Can you work these out from the drawing? Everything is in mm from the part's minimum corner. Round coordinates to 2 decimals unless told otherwise and drop trailing zeros. Loops run counter-clockwise (first coordinate to the right, second up) from the corner with the lowest first, then second, coordinate; pieces in that order, holes last. Notation, with made-up numbers: (24, 80.5) - (69, 80.5) arc R21 ccw to (69, 98.5) - close; hole circle Ø10 at (-27, 45.5). An arc over 180 degrees is marked (long way). Answer as a JSON object with one key per item and string values. Group by question number.
1) I want a section at C-C, the plane y = 28. Please give me the cut outline in (x, z).
2) I want a section at B-B, the plane x = 1.1. Please give me the cut outline in (y, z).
3) I want a section at A-A, the plane z = 27. Please give me the cut outline in (x, y).
4) If I drill on line 1 along Y through (x, z) = (0.5, 3); line 2 along Z through (x, y) = (0.3, 3.5); line 3 along Y through (x, z) = (0.15, 28.5), over which ranges is the centre line in solid material (lowest first)? Write a range as [from, to].
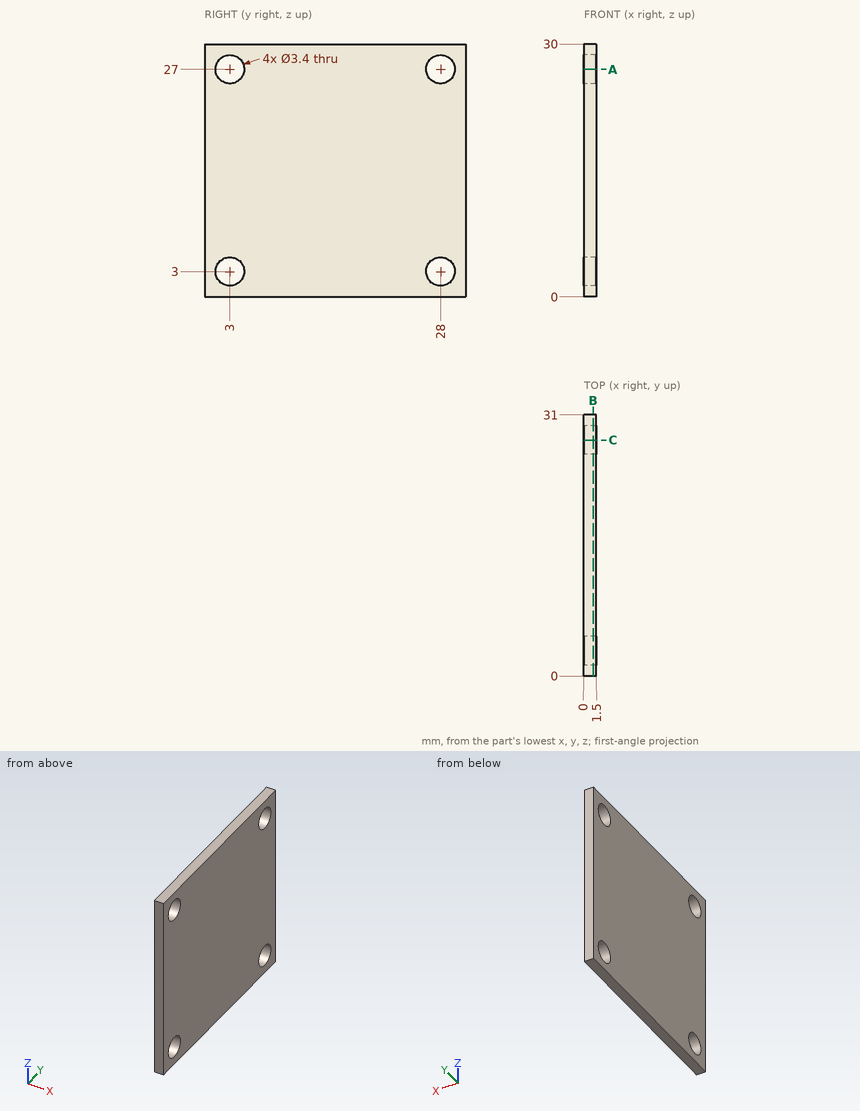
Outcome:
{
 "1": {"outline": "(0, 0) - (1.5, 0) - (1.5, 1.3) - (0, 1.3) - close; (0, 4.7) - (1.5, 4.7) - (1.5, 25.3) - (0, 25.3) - close; (0, 28.7) - (1.5, 28.7) - (1.5, 30) - (0, 30) - close"},
 "2": {"outline": "(0, 0) - (31, 0) - (31, 30) - (0, 30) - close; hole circle Ø3.4 at (3, 3); hole circle Ø3.4 at (3, 27); hole circle Ø3.4 at (28, 3); hole circle Ø3.4 at (28, 27)"},
 "3": {"outline": "(0, 0) - (1.5, 0) - (1.5, 1.3) - (0, 1.3) - close; (0, 4.7) - (1.5, 4.7) - (1.5, 26.3) - (0, 26.3) - close; (0, 29.7) - (1.5, 29.7) - (1.5, 31) - (0, 31) - close"},
 "4": {"line 1": "[0, 1.3], [4.7, 26.3], [29.7, 31]", "line 2": "[0, 1.38], [4.62, 25.38], [28.62, 30]", "line 3": "[0, 2.2], [3.8, 27.2], [28.8, 31]"}
}
